from build123d import *

# Parameters (mm, degrees)
F0_R     = 19.05
F0_R_2   = 5.000003
F1_DEPTH = 177.8
F2_R     = 10.000005
F3_DEPTH = 12.999999
F4_SIZE  = 2.54


with BuildPart() as f1:
    # F0 (on Top) → F1 (new body)
    with BuildSketch(Plane.XY):
        Circle(F0_R)
        Circle(F0_R_2, mode=Mode.SUBTRACT)
    extrude(amount=F1_DEPTH)

    # F2 (on Top) → F3 (join)
    with BuildSketch(Plane.XY):
        Polygon((5.886217, -18.115914), (19.048199, 0), (5.886217, 18.115914), (-15.410317, 11.19625), (-15.410317, -11.19625), align=None)
        Circle(F2_R, mode=Mode.SUBTRACT)
    extrude(amount=-F3_DEPTH)

    # F4
    f4_edges = [f1.edges().sort_by_distance(p)[0] for p in [
        (-19.05, 0, 177.8),
    ]]
    chamfer(f4_edges, length=F4_SIZE)


solid = f1.part
Verification items for the finished model (mm, model axes). A direction names the side the tool comes from. Round coordinates to 2 decimals unless told otherwise and drop trailing zeros. Loops run counter-clockwise (first coordinate to the right, second up) from the corner with the lowest first, then second, coordinate; pieces in that order, holes last. Notation, with made-up numbers: (30.25, 49) - (80.25, 49) arc R8 ccw to (80.25, 62) - close; hole circle Ø8 at (1.5, 28.25). An arc over 180 degrees is marked (long way). Use a Markdown table: item, result. Add a question column.
1. Thickness scan on probe 1 along Y at (x, z) = (0, 87); probe 2 along X at (y, z) = (3.5, 145); probe 3 along Z at (x, y) = (-7, 5). Record the ranges inside material, lowest first. Write a range as [from, to].
2. Section check A-A, the plane x = 0. Record the boundary of the cut face in (y, z), plus the area to 3 significant figures.
3. Release check for a two-part mould opening along X. For faces 1 (the face through (-4.613, 14.705, -6.409)), 2 (the face through (12.56, 8.93, -6.41)), 3 (the face through (-0.651, 4.957, 87.655)) record: released by +X, released by -X, zero draft, split by the parting line, or undercut.
4. Access from +Z, -Z, +X, -X, +Y, -Y to the whole of each face (thin tool, end or side, straight path). Record for faces 4 (the face through (-15.41, 0, -6)), 5 (the face through (12.38, -9.18, -6.41)), 6 (the face through (-2.17, -9.76, -6.41)).
5. Section check B-B, the plane z = 67.5. Record the boundary of the cut face in (x, y).
6. Gauge pin test, flat ends, axial feed: pin 1 (12 mm diameter, centred on x = -12, z = 58, fed in from -Y); pin 2 (4 mm diameter, centred on y = 4.5, z = -3.5, fed in from -X); pin 3 (3 mm diameter, centred on x = 1.5, z = 131, fed in from +Y); pin 4 (18 mm diameter, centred on x = 0, y = 0, fed in from +Z). Record the tip position at first contact, or that the pin passes through.
Checks:
| question | item | result |
|---|---|---|
| 1 | probe 1 | y = [-19.05, -5], [5, 19.05] |
| 1 | probe 2 | x = [-18.73, -3.57], [3.57, 18.73] |
| 1 | probe 3 | z = [0, 177.8] |
| 2 | outline | (-19.05, 0) - (-16.2, 0) - (-16.2, -13) - (-10, -13) - (-10, 0) - (-5, 0) - (-5, 177.8) - (-16.51, 177.8) - (-19.05, 175.26) - close; (5, 0) - (10, 0) - (10, -13) - (16.2, -13) - (16.2, 0) - (19.05, 0) - (19.05, 175.26) - (16.51, 177.8) - (5, 177.8) - close |
| 2 | area | 5,150 mm^2 |
| 3 | face 1 | released by -X |
| 3 | face 2 | released by +X |
| 3 | face 3 | undercut |
| 4 | face 4 | -Z, -X, +Y, -Y |
| 4 | face 5 | -Z, +X, -Y |
| 4 | face 6 | -Z |
| 5 | outline | circle Ø38.1 at (0, 0); hole circle Ø10 at (0, 0) |
| 6 | pin 1 | stops at y = -18.08 |
| 6 | pin 2 | stops at x = -15.41 |
| 6 | pin 3 | stops at y = 19.05 |
| 6 | pin 4 | stops at z = 177.8 |
